The listing builds one solid part. Answer for the finished solid, in the listing's coordinates (mm). A direction names the side the tool comes from. Give positions to 0.01 mm unless a question says otherwise; leave off trailing zeros. Loops run counter-clockwise (first coordinate to the right, second up) from the corner with the lowest first, then second, coordinate; pieces in that order, holes last. Notation, with made-up numbers: M 7,-15 L 43,-15 A13 ccw 43,0 Z; hole C 47,-6.5 d11. An arc over 180 degrees is marked long. One line per item, written item: value. Start each with the question number.
Q1. A cutting plane is placed at B-B, the plane y = 29.5. Determine the outline of the cut face in (x, z), and give its area (3 significant figures).
Q2. Flat-ended cylindrical pins translate along their axes: pin 1 (10 mm diameter, centred on x = 141.5, z = 7.5, fed in from -Y); pin 2 (12.5 mm diameter, centred on x = 41, y = 37, fed in from +Z); pin 3 (3 mm diameter, centred on x = 115, y = 22, fed in from -Z). Find the tip coordinate at first contact, or state that the pin passes through.
Q3. For faces 1 (the flat face through (50, 44, -20)), 2 (the flat face through (50, 45, 20)), 3 (the flat face through (50, 5, 19)), determine the directions among +Z, -Z, +X, -X, +Y, -Y from which every point of the face is accessible in a straight line to the end or side of a thin tool.
Q4. A cutting plane is placed at C-C, the plane z = 19. Determine the outline of the cut face in (x, y).
Q5. A cutting plane is placed at D-D, the plane x = 86.5. Determine the outline of the cut face in (y, z).
Q6. A cutting plane is placed at A-A, the plane x = 0. Determine the outline of the cut face in (y, z), and give its area (3 significant figures).
Q7. Consider L1, parallel to X at y = 20, z = 0; L2, parallel to X at y = 11, z = 165.5; L3, parallel to Z at x = -6, y = 8. Determine where each line is inside the solid, lowest interval first.
from build123d import *

# Parameters (mm, degrees)
BOSS_EXTRUDE2_DEPTH = 50
SKETCH2_R           = 10
CUT_EXTRUDE1_DEPTH  = 189.745860882
SKETCH3_R           = 25
BOSS_EXTRUDE3_DEPTH = 200


with BuildPart() as part:
    # Sketch1 → Boss-Extrude2 (new body)
    with BuildSketch(Plane(origin=(0, 0, 0), x_dir=(1, 0, 0), z_dir=(0, 1, 0))):
        Polygon((-25, 25), (25, 25), (50, 25), (50, -25), (25, -25), (25, -175), (-25, -175), align=None)
    extrude(amount=BOSS_EXTRUDE2_DEPTH)

    # Sketch2 → Cut-Extrude1 (cut, through all)
    with BuildSketch(Plane.XZ):
        with Locations(Location((0, 0, 0), (0, 0, 270))):
            Circle(SKETCH2_R)
    extrude(amount=-CUT_EXTRUDE1_DEPTH, mode=Mode.SUBTRACT)

    # Sketch3 → Boss-Extrude3 (add)
    with BuildSketch(Plane(origin=(50, 0, 0), x_dir=(0, 0, -1), z_dir=(1, 0, 0))):
        with Locations((0, 25)):
            Circle(SKETCH3_R)
    extrude(amount=BOSS_EXTRUDE3_DEPTH)


solid = part.part
Answer block:
1. outline: M -25,-25 L 50,-25 L 50,-24.59 L 250,-24.59 L 250,24.59 L 50,24.59 L 50,25 L 25,25 L 25,175 L -25,175 Z; hole C 0,0 d20
1. area: 20,800 mm^2
2. pin 1: y = 0.13
2. pin 2: z = 25
2. pin 3: z = -24.95
3. face 1: -Z, +X, +Y
3. face 2: +Z, +X, +Y
3. face 3: +Z, +X, -Y
4. outline: M -25,0 L 50,0 L 50,8.75 L 250,8.75 L 250,41.25 L 50,41.25 L 50,50 L -25,50 Z
5. outline: C 25,0 d50
6. outline: M 0,-25 L 50,-25 L 50,-10 L 0,-10 Z; M 0,10 L 50,10 L 50,175 L 0,175 Z
6. area: 9,000 mm^2
7. L1: -25 to -10, 10 to 250
7. L2: -25 to 25
7. L3: -25 to -8, 8 to 175
